```python
from build123d import *

# Parameters (mm, degrees)
EXTRUDE_1_DEPTH      = 3
M3X0_5_1_D           = 2.5
M3X0_5_1_CSINK_D     = 3.05
M3X0_5_1_CSINK_ANGLE = 90
FILLET_1_R           = 0.6


with BuildPart() as part:
    # 草图1 → 凸台-拉伸1 (new body)
    with BuildSketch(Plane.XY):
        with BuildLine():
            Line((6, 4.5), (30, 4.5))
            ThreePointArc((30, 4.5), (31.414213562, 3.914213562), (32, 2.5))
            Line((32, 2.5), (32, -2.5))
            ThreePointArc((32, -2.5), (31.414213562, -3.914213562), (30, -4.5))
            Line((30, -4.5), (6, -4.5))
            ThreePointArc((6, -4.5), (0, -7.5), (-6, -4.5))
            Line((-6, -4.5), (-30, -4.5))
            ThreePointArc((-30, -4.5), (-31.414213562, -3.914213562), (-32, -2.5))
            Line((-32, -2.5), (-32, 2.5))
            ThreePointArc((-32, 2.5), (-31.414213562, 3.914213562), (-30, 4.5))
            Line((-30, 4.5), (-6, 4.5))
            ThreePointArc((-6, 4.5), (-3.045393494, 6.853873246), (0.681818182, 7.468943966))
            ThreePointArc((0.681818182, 7.468943966), (3.6558625, 6.548638742), (6, 4.5))
        make_face()
        with BuildLine():
            Line((0.6, 7.275300681), (0.6, 2.375394704))
            ThreePointArc((0.6, 2.375394704), (1.385836512, 2.020385399), (2, 1.41509717))
            Line((2, 1.41509717), (2, -1.41509717))
            ThreePointArc((2, -1.41509717), (-2.020385399, -1.385836512), (-0.6, 2.375394704))
            Line((-0.6, 2.375394704), (-0.6, 7.275300681))
            ThreePointArc((-0.6, 7.275300681), (0, 7.3), (0.6, 7.275300681))
        make_face(mode=Mode.SUBTRACT)
    extrude(amount=EXTRUDE_1_DEPTH)

    # M3x0.5 螺纹孔1 (through all)
    with Locations(Plane.XY.offset(3)):
        with Locations((-29, 0), (29, 0)):
            CounterSinkHole(M3X0_5_1_D / 2, M3X0_5_1_CSINK_D / 2, counter_sink_angle=M3X0_5_1_CSINK_ANGLE)

    # 圆角1
    fillet_1_edges = [part.edges().sort_by_distance(p)[0] for p in [
        (0.6, 7.275300681, 1.5),
        (-0.6, 7.275300681, 1.5),
        (2, -1.41509717, 1.5),
        (2, 1.41509717, 1.5),
        (-6, -4.5, 1.5),
        (6, -4.5, 1.5),
        (6, 4.5, 1.5),
        (-6, 4.5, 1.5),
    ]]
    fillet(fillet_1_edges, radius=FILLET_1_R - 0.0001)  # a hair under: the kernel refuses the full size


solid = part.part
```
For this review, take the finished solid that the model builds, in its own axes (mm). A direction names the side the tool comes from. Round coordinates to 2 decimals unless told otherwise and drop trailing zeros. Order: outer loops, then holes, each group sorted by start corner. A loop starts at its lowest first (then second) coordinate and runs counter-clockwise, first axis right, second up. Notation, with made-up numbers: (73.5, -2.5) -> (92.5, -2.5) arc R16 cw to (92.5, 15.5) -> close; hole circle Ø3 at (37, 43). An arc over 180 degrees is marked (long way). Use a Markdown table: item, result.
Item 1: Take a section at D-D (y = 5.25). State the section outline as (x, z) points, plus the area to 3 significant figures.
Resolved:
| item | result |
|---|---|
| outline | (-5.36, 0) -> (-0.6, 0) -> (-0.6, 3) -> (-5.36, 3) -> close; (0.6, 0) -> (5.36, 0) -> (5.36, 3) -> (0.6, 3) -> close |
| area | 28.5 mm² |
Item 2: For line 1 along X through (y, z) = (0, 0.6); line 2 along Y through (x, z) = (-29, 2.25); line 3 along Y through (x, z) = (-11, 1.15), list the stretches that pass through material, from the lowest coordinate up. Write a range as [from, to].
Resolved:
| item | result |
|---|---|
| line 1 | x = [-32, -30.25], [-27.75, -2.45], [2, 27.75], [30.25, 32] |
| line 2 | y = [-4.5, -1.25], [1.25, 4.5] |
| line 3 | y = [-4.5, 4.5] |
Item 3: Take a section at A-A (x = -29). State the section outline as (y, z) points (3 decimals), plus the area to 3 significant figures.
Resolved:
| item | result |
|---|---|
| outline | (-4.5, 0) -> (-1.25, 0) -> (-1.25, 2.725) -> (-1.525, 3) -> (-4.5, 3) -> close; (1.25, 0) -> (4.5, 0) -> (4.5, 3) -> (1.525, 3) -> (1.25, 2.725) -> close |
| area | 19.4 mm² |
Item 4: For pin 1 (0.9 mm diameter, centred on x = 14, z = 1.5, fed in from +Y); pin 2 (0.9 mm diameter, centred on x = -23, z = 2, fed in from -Y); pin 3 (1.5 mm diameter, centred on y = 5.5, z = 1.5, fed in from +X), all flat-tipped, find the tip position at first contact; note any pin that passes through.
Resolved:
| item | result |
|---|---|
| pin 1 | stops at y = 4.5 |
| pin 2 | stops at y = -4.5 |
| pin 3 | stops at x = 5.8 |
Item 5: Take a section at C-C (z = 1.15). State how many separate pieces and enclosed holes the cut face has, plus the area to 3 significant figures.
Resolved:
| item | result |
|---|---|
| separate pieces | 1 |
| enclosed holes | 3 |
| area | 589 mm² |
Item 6: Take a section at B-B (y = 0). State the section outline as (x, z) points (3 decimals).
Resolved:
| item | result |
|---|---|
| outline | (-32, 0) -> (-30.25, 0) -> (-30.25, 2.725) -> (-30.525, 3) -> (-32, 3) -> close; (-27.75, 0) -> (-2.45, 0) -> (-2.45, 3) -> (-27.475, 3) -> (-27.75, 2.725) -> close; (2, 0) -> (27.75, 0) -> (27.75, 2.725) -> (27.475, 3) -> (2, 3) -> close; (30.25, 0) -> (32, 0) -> (32, 3) -> (30.525, 3) -> (30.25, 2.725) -> close |
Item 7: Machinability: for faces 1 (the flat face through (-18, 4.5, 1)), 2 (the flat face through (18, 4.5, 1)), 3 (the flat face through (-0.6, 5, 1)), which of the approach directions +Z, -Z, +X, -X, +Y, -Y give a long, thin tool a straight path to every point of the face, cutting with its end or side? Answer none if there is none.
Resolved:
| item | result |
|---|---|
| face 1 | +Z, -Z, -X, +Y |
| face 2 | +Z, -Z, +X, +Y |
| face 3 | +Z, -Z |
Item 8: Draft analysis for pull direction X (two halves, no side actions). For faces 4 (the flat face through (0, -3, 3)), 5 (the flat face through (32, 0, 1)), 6 (the cylindrical face through (1.28, 2.09, 1.48)), state which applies: +X half, -X half, draft (parallel to the pull), parting line (faces both ways), or undercut.
Resolved:
| item | result |
|---|---|
| face 4 | draft |
| face 5 | +X half |
| face 6 | undercut |
